Geometry check sheet. Reference: the model listing, model coordinates, mm. Coordinates: 2 decimals unless noted, no trailing zeros. Order: outer loops, then holes, each group sorted by start corner. A loop starts at its lowest first (then second) coordinate and runs counter-clockwise, first axis right, second up. Notation, with made-up numbers: M -24.5,49 L 25.5,49 A23 ccw 25.5,67 Z; hole C 2.5,14 d10. An arc over 180 degrees is marked long. One line per item, written item: value. Start each with the question number.
1) Sectioned sample at D-D, the plane x = -30.5. Enter the section's corners in (y, z).
2) Draft check along X on faces 1 (the cylindrical face through (0.18, 40.705, 3.451)), 2 (the flat face through (-11, -3, 0)), 3 (the cylindrical face through (-13.24, -17.99, 3.45)). Enter one of: pulls with the +X half, pulls with the -X half, needs draft (parallel to the pull), parting line crosses it, or undercut.
3) Go/stop test with flat-tipped pins: P1, Ø4, axis at y = -3.5, z = 5.5, coming from the +X side; P2, Ø4, axis at y = 8, z = 1.5, coming from the +X side; P3, Ø2, axis at y = 31, z = 1, coming from the +X side; P4, Ø5, axis at x = -17, y = 1.5, coming from the +Z side. Record where each tip stops, or that it passes through.
4) Sectioned sample at B-B, the plane y = 35. Enter the section's corners in (x, z), then the cut area to 3 significant figures.
5) Sectioned sample at A-A, the plane x = -2. Enter the section's corners in (y, z), then the cut area to 3 significant figures.
6) Thickness scan on L1, parallel to Y at x = 0, z = 4.75; L2, parallel to Y at x = 9, z = 3.25; L3, parallel to X at y = 27, z = 2. Record the ranges inside material, lowest first. Write a range as from..to.
7) Sectioned sample at C-C, the plane z = 2.25. Enter the section's corners in (x, y), then the cut area to 3 significant figures.
```python
from build123d import *

# Parameters (mm, degrees)
F0_R     = 11.2
F1_DEPTH = 7


with BuildPart() as f1:
    # F0 (on Top) → F1 (new body)
    with BuildSketch(Plane.XY):
        with BuildLine():
            ThreePointArc((20.649142, -0.505374), (11.268043, 6.660297), (10.250514, 18.421101))
            ThreePointArc((10.250514, 18.421101), (-0.25463, 40.703741), (-9.911882, 18.040741))
            ThreePointArc((-9.911882, 18.040741), (-11.426986, 6.333635), (-21.103376, -0.427973))
            ThreePointArc((-21.103376, -0.427973), (-35.148137, -20.667014), (-10.692777, -17.69894))
            ThreePointArc((-10.692777, -17.69894), (0.203426, -13.157505), (10.897346, -18.156701))
            ThreePointArc((10.897346, -18.156701), (35.44725, -20.2003), (20.649142, -0.505374))
        make_face()
        with Locations((-23.586189, -13.697699)):
            Circle(F0_R, mode=Mode.SUBTRACT)
        Circle(F0_R, mode=Mode.SUBTRACT)
        with Locations((23.630672, -13.672017)):
            Circle(F0_R, mode=Mode.SUBTRACT)
        with Locations((0, 27.206143)):
            Circle(F0_R, mode=Mode.SUBTRACT)
    extrude(amount=F1_DEPTH)


solid = f1.part
```
Final values:
1. outline: M -25.29,0 L -22.51,0 L -22.51,7 L -25.29,7 Z; M -4.89,0 L -2.1,0 L -2.1,7 L -4.89,7 Z
2. face 1: parting line crosses it
2. face 2: needs draft
2. face 3: undercut
3. P1: stops at x = 34.38
3. P2: stops at x = 11.65
3. P3: stops at x = 13.21
3. P4: stops at z = 7
4. outline: M -11.02,0 L -8.04,0 L -8.04,7 L -11.02,7 Z; M 8.04,0 L 11.02,0 L 11.02,7 L 8.04,7 Z
4. area: 41.7 mm^2
5. outline: M -13.28,0 L -11.02,0 L -11.02,7 L -13.28,7 Z; M 11.02,0 L 16.19,0 L 16.19,7 L 11.02,7 Z; M 38.23,0 L 40.56,0 L 40.56,7 L 38.23,7 Z
5. area: 68.3 mm^2
6. L1: y = -13.15..-11.2, 11.2..16.01, 38.41..40.71
6. L2: y = -16.34..-6.67, 6.67..20.54, 33.87..37.27
6. L3: x = -13.5..-11.2, 11.2..13.5
7. outline: M -21.1,-0.43 A13.5 ccw long -10.69,-17.7 A14.6 cw 10.9,-18.16 A13.5 ccw long 20.65,-0.51 A14.6 cw 10.25,18.42 A13.5 ccw long -9.91,18.04 A14.6 cw Z; hole C -23.59,-13.7 d22.4; hole C 0,0 d22.4; hole C 0,27.21 d22.4; hole C 23.63,-13.67 d22.4
7. area: 870 mm^2
